```python
from build123d import *

# Parameters (mm, degrees)
SKETCH1_W             = 54.45
SKETCH1_H             = 20
BOSS_EXTRUDE1_DEPTH   = 3.175
BOSS_EXTRUDE2_DEPTH   = 54.45
SKETCH3_W             = 25.4
SKETCH3_H             = 31.43
BOSS_EXTRUDE3_DEPTH   = 3.175
CHAMFER1_SIZE         = 1.5875
CHAMFER2_SIZE         = 12.7
SKETCH5_W             = 31.75
SKETCH5_H             = 31.43
BOSS_EXTRUDE5_DEPTH   = 4.7498
CHAMFER3_SIZE         = 12.7
CHAMFER4_SIZE         = 1.5875
F_6_CLEARANCE_HOLE1_D = 4.3053


with BuildPart() as part:
    # Sketch1 → Boss-Extrude1 (new body)
    with BuildSketch(Plane.XY):
        with Locations((29.025, 8.610649597)):
            Rectangle(SKETCH1_W, SKETCH1_H)
    extrude(amount=BOSS_EXTRUDE1_DEPTH)

    # Sketch2 → Boss-Extrude2 (add)
    with BuildSketch(Plane(origin=(56.25, 0, 0), x_dir=(0, 0, -1), z_dir=(1, 0, 0))):
        Polygon((0, 18.610649597), (0, 21.150649597), (22.225, 21.150649597), (22.225, 24.325649597), (-3.175, 24.325649597), (-3.175, 18.610649597), align=None)
        Polygon((22.225, -3.929350403), (22.225, -7.104350403), (-3.175, -7.104350403), (-3.175, -1.389350403), (0, -1.389350403), (0, -3.929350403), align=None)
    extrude(amount=-BOSS_EXTRUDE2_DEPTH)

    # Sketch3 → Boss-Extrude3 (add)
    with BuildSketch(Plane(origin=(56.25, 0, 0), x_dir=(0, 0, -1), z_dir=(1, 0, 0))):
        with Locations((9.525, 8.610649597)):
            Rectangle(SKETCH3_W, SKETCH3_H)
    extrude(amount=BOSS_EXTRUDE3_DEPTH)

    # Chamfer1
    chamfer1_edges = [part.edges().sort_by_distance(p)[0] for p in [
        (29.025, 21.150649597, 0),
        (56.25, 21.150649597, -11.1125),
        (29.025, -3.929350403, 0),
        (56.25, -3.929350403, -11.1125),
        (59.425, 8.610649597, 3.175),
        (59.425, -7.104350403, -9.525),
        (59.425, 24.325649597, -9.525),
        (56.25, 8.610649597, 0),
    ]]
    chamfer(chamfer1_edges, length=CHAMFER1_SIZE)

    # Chamfer2
    chamfer2_edges = [part.edges().sort_by_distance(p)[0] for p in [
        (1.8, 22.738149597, -22.225),
        (1.8, -5.516850403, -22.225),
    ]]
    chamfer(chamfer2_edges, length=CHAMFER2_SIZE)

    # Sketch5 → Boss-Extrude5 (add)
    with BuildSketch(Plane.XY.offset(3.175)):
        with Locations((17.675, 8.610649597)):
            Rectangle(SKETCH5_W, SKETCH5_H)
    extrude(amount=BOSS_EXTRUDE5_DEPTH)

    # Chamfer3
    # the kernel refuses this chamfer: 12.7 mm, written as the material it adds along each edge
    with BuildSketch(Plane(origin=(33.55, 24.325649597, 3.175), x_dir=(0.9996219169112966, 0, -0.02749587661058638), z_dir=(0, -1, 0))) as chamfer3_piece_1_section:
        Polygon((CHAMFER3_SIZE * 0.999621916911, CHAMFER3_SIZE * 0.0274958766106), (-CHAMFER3_SIZE * 0.0274958766106, CHAMFER3_SIZE * 0.999621916911), (0, 0), align=None)
    chamfer3_piece_1 = extrude(amount=31.43, mode=Mode.PRIVATE)
    chamfer3_piece_1 = split(chamfer3_piece_1, bisect_by=Plane(origin=(38.87834153, 8.610649597, 7.9248), z_dir=(0, 0, -1)), keep=Keep.TOP, mode=Mode.PRIVATE)
    add(chamfer3_piece_1)

    # Chamfer4
    chamfer4_edges = [part.edges().sort_by_distance(p)[0] for p in [
        (21.6501, 24.325649597, 7.9248),
        (21.6501, -7.104350403, 7.9248),
        (1.8, 8.610649597, 7.9248),
        (52.04375, -7.104350403, 3.175),
        (52.04375, 24.325649597, 3.175),
        (43.8751, 24.325649597, 5.5499),
        (43.8751, -7.104350403, 5.5499),
    ]]
    chamfer(chamfer4_edges, length=CHAMFER4_SIZE)

    # #6 Clearance Hole1 (through all)
    with Locations(Plane.XY.offset(7.9248)):
        with Locations((10, 12.610649597), (30, 4.610649597)):
            Hole(F_6_CLEARANCE_HOLE1_D / 2)


solid = part.part
```
Model file for the job. Use its own axes, mm. A direction names the side the tool comes from. Coordinates: 2 decimals unless noted, no trailing zeros. Loops run counter-clockwise (first coordinate to the right, second up) from the corner with the lowest first, then second, coordinate; pieces in that order, holes last. Notation, with made-up numbers: (55.5, 5) -> (61.5, 5) arc R31 ccw to (61.5, 44) -> close; hole circle Ø1 at (55, 45.5). An arc over 180 degrees is marked (long way). Answer as a JSON object with one key per item and string values.
Q1. Probe probe 1 along Y at (x, z) = (30, 4); probe 2 along Y at (x, z) = (28.5, -2); probe 3 along X at (y, z) = (6, -10.5) (3 decimals). List the from-to ranges inside material, lowest first.
Report:
{"probe 1": "y = -7.1 to 2.46, 6.76 to 24.33", "probe 2": "y = -7.1 to -3.93, 21.15 to 24.33", "probe 3": "x = 56.25 to 59.425"}
Q2. Cut at D-D (z = 4). List the corners of the cut face in (x, y) (3 decimals).
Report:
{"outline": "(1.8, -7.104) -> (43.18, -7.104) -> (45.425, -5.517) -> (45.425, 22.738) -> (43.18, 24.326) -> (1.8, 24.326) -> close; hole circle Ø4.305 at (10, 12.611); hole circle Ø4.305 at (30, 4.611)"}
Q3. Pull direction Y, two halves, no side cores. Call faces 1 (the cylindrical face through (10.28, 14.745, 3.907)), 2 (the flat face through (8.239, 22.716, -15.964)), 3 (the flat face through (52.02, -6.32, 2.37)), 4 (the flat face through (55.269, -2.844, -1.108)): released by +Y, released by -Y, zero draft, split by the parting line, or undercut.
Report:
{"face 1": "undercut", "face 2": "zero draft", "face 3": "released by -Y", "face 4": "undercut"}
Q4. Flat gauge pins, fed straight in: P1, Ø6.5, axis at x = 16, y = 10, coming from the -Z side; P2, Ø5, axis at y = 8.5, z = -5, coming from the -X side; P3, Ø9.5, axis at x = 53.5, y = 2.5, coming from the +Z side (3 decimals); P4, Ø3.5, axis at x = 10, y = 12.61, coming from the +Z side. Where does each tip first touch, or does it go through?
Report:
{"P1": "stops at z = 0", "P2": "stops at x = 56.25", "P3": "stops at z = 3.175", "P4": "passes through"}
Q5. 3-axis set-ups, long thin cutter, end or side, ignore diameter. For faces 5 (the flat face through (59.425, 9, -10)), 6 (the flat face through (52, 8, 3.175)), 7 (the flat face through (55.467, 8.764, -0.805)): which of +Z, -Z, +X, -X, +Y, -Y reach the whole face in a straight line?
Report:
{"face 5": "+Z, -Z, +X, +Y, -Y", "face 6": "+Z, +X, +Y, -Y", "face 7": "-Z, -X"}
Q6. Cut at A-A (x = 30). List the corners of the cut face in (y, z) (1 decimal), and give its area (3 significant figures).
Report:
{"outline": "(-7.1, -22.2) -> (-3.9, -22.2) -> (-3.9, -1.6) -> (-2.3, 0) -> (2.5, 0) -> (2.5, 7.9) -> (-5.5, 7.9) -> (-7.1, 6.3) -> close; (6.8, 0) -> (19.6, 0) -> (21.2, -1.6) -> (21.2, -22.2) -> (24.3, -22.2) -> (24.3, 6.3) -> (22.7, 7.9) -> (6.8, 7.9) -> close", "area": "356 mm2"}
